```python
from build123d import *

# Parameters (mm, degrees)
SKETCH3_R                = 1.6
BOSS_EXTRUDE2_DEPTH      = 5
SKETCH8_W                = 6.531662429
SKETCH8_H                = 15.718756423
BOSS_EXTRUDE5_DEPTH      = 25.594989388
BOSS_EXTRUDE6_DEPTH      = 5
BOSS_EXTRUDE6_DEPTH_BACK = 15.725319597
BOSS_EXTRUDE7_DEPTH      = 15.715206985
FILLET3_R                = 6


with BuildPart() as part:
    # Sketch3 → Boss-Extrude2 (new body)
    with BuildSketch(Plane.XY):
        with BuildLine():
            Line((15.398328751, 23.358235096), (42.103650237, 35.3480109))
            ThreePointArc((42.103650237, 35.3480109), (43.812929052, 35.351800988), (44.957199874, 34.082040099))
            Line((44.957199874, 34.082040099), (42.962535727, 10.043789437))
            ThreePointArc((42.962535727, 10.043789437), (39.652134692, -17.353336053), (40.589325164, -44.933816726))
            Line((40.589325164, -44.933816726), (46.4215305, -44.933816726))
            Line((46.4215305, -44.933816726), (46.4215305, -60.652573149))
            Line((46.4215305, -60.652573149), (28.574574678, -60.652573149))
            ThreePointArc((28.574574678, -60.652573149), (27.026794649, -59.729266605), (26.047291344, -58.216424488))
            ThreePointArc((26.047291344, -58.216424488), (16.153529465, -18.922365583), (14.162802755, 21.549187347))
            ThreePointArc((14.162802755, 21.549187347), (14.525551977, 22.627878073), (15.398328751, 23.358235096))
        make_face()
        with Locations((17.26515434, 20.395199458)):
            Circle(SKETCH3_R, mode=Mode.SUBTRACT)
        with Locations((41.82515434, 31.625199458)):
            Circle(SKETCH3_R, mode=Mode.SUBTRACT)
        with Locations((39.04515434, 14.855199458)):
            Circle(SKETCH3_R, mode=Mode.SUBTRACT)
    extrude(amount=BOSS_EXTRUDE2_DEPTH)

    # Sketch8 → Boss-Extrude5 (add)
    with BuildSketch(Plane.XY.offset(5)):
        with Locations((43.155699286, -52.793194938)):
            Rectangle(SKETCH8_W, SKETCH8_H)
    extrude(amount=BOSS_EXTRUDE5_DEPTH)

    # Sketch9 → Boss-Extrude6 (add, two sides: drawn at the far end of the back side and taken through both)
    with BuildSketch(Plane(origin=(0, -44.933816726, 0), x_dir=(1, 0, 0), z_dir=(0, 1, 0)).offset(-BOSS_EXTRUDE6_DEPTH_BACK)):
        with BuildLine():
            Line((46.4215305, -30.594989388), (46.4215305, 0))
            Line((46.4215305, 0), (46.4215305, 2.879605598))
            Line((46.4215305, 2.879605598), (50.894134372, 2.879605598))
            ThreePointArc((50.894134372, 2.879605598), (48.34293367, -13.815617676), (46.4215305, -30.594989388))
        make_face()
    extrude(amount=BOSS_EXTRUDE6_DEPTH + BOSS_EXTRUDE6_DEPTH_BACK)

    # Sketch10 → Boss-Extrude7 (add)
    with BuildSketch(Plane(origin=(0, -44.933816726, 0), x_dir=(1, 0, 0), z_dir=(0, 1, 0))):
        with BuildLine():
            Line((29.146955031, -5), (41.859352304, -5))
            Line((41.859352304, -5), (41.859352304, -30.594989388))
            ThreePointArc((41.859352304, -30.594989388), (38.401030969, -16.358190815), (29.146955031, -5))
        make_face()
    extrude(amount=-BOSS_EXTRUDE7_DEPTH)

    # Fillet3
    # the kernel refuses this fillet: 6 mm, written as the material it adds along each edge
    with BuildSketch(Plane(origin=(46.4215305, -44.933816726, 30.594989388), x_dir=(0, 1, 0), z_dir=(0, 0, -1))) as fillet3_piece_1_section:
        with BuildLine():
            CenterArc((6, -5.916079783), FILLET3_R, 99.594068227, 80.405931773)
            Line((0, -5.916079783), (-0.12, -5.916079783))
            Line((-0.12, -5.916079783), (-0.12, 0))
            Line((-0.12, 0), (0, 0.12))
            ThreePointArc((0, 0.12), (2.5, 0.12), (4.98, 0.118321596))
            Line((4.98, 0.118321596), (5, 0))
        make_face()
    fillet3_piece_1 = extrude(amount=30.594989388, mode=Mode.PRIVATE)
    fillet3_piece_1 = fillet3_piece_1 - Plane(origin=(493.305440786, -43.701646152, 73.26789881), x_dir=(-0.9855086772136745, 0, -0.16962501919396705), z_dir=(0, -1, 0)) * Cylinder(448.916703265, 85, mode=Mode.PRIVATE)
    add(fillet3_piece_1)


solid = part.part
```
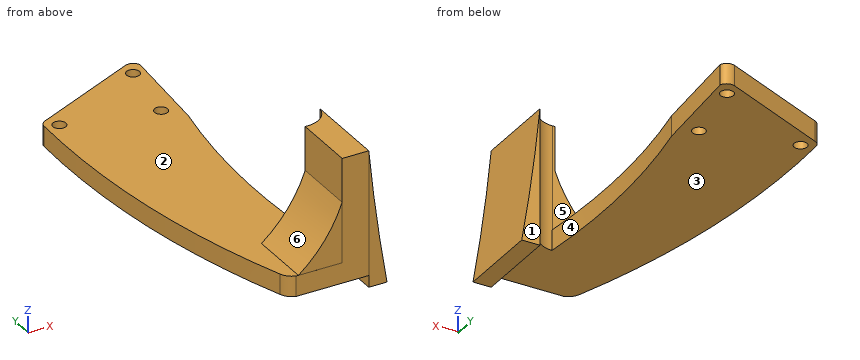
Input: part model. Units: mm. Frame: model coordinates. Face numbers are marked on the shaded views. A direction names the side the tool comes from. Round coordinates to 2 decimals unless told otherwise and drop trailing zeros. Loops run counter-clockwise (first coordinate to the right, second up) from the corner with the lowest first, then second, coordinate; pieces in that order, holes last.
1) Section query A-A on z = 1. Count the separate pieces of the cut face and the enclosed holes in it, plus the area to 3 significant figures.
Ans:
separate pieces: 1
enclosed holes: 3
area: 2,300 mm2
2) Pin query (flat end, axial travel): pin 1 (1.5 mm diameter, centred on x = 37, z = 10, fed in from -Y); pin 2 (5 mm diameter, centred on x = 41.83, y = 31.63, fed in from -Z); pin 3 (10 mm diameter, centred on x = 36, z = 3, fed in from -Y). Return the tip coordinate at first contact, or that it passes through.
Ans:
pin 1: stops at y = -60.65
pin 2: stops at z = 0
pin 3: stops at y = -60.65
3) Section query D-D on y = -51. Return the cut outline in (x, z), plus the area to 3 significant figures.
Ans:
outline: (23.6, 0) - (46.42, 0) - (46.42, -2.88) - (50.89, -2.88) arc R448.92 cw to (46.42, 30.59) - (39.89, 30.59) - (39.89, 19.84) arc R33.17 cw to (29.15, 5) - (23.6, 5) - close
area: 413 mm2
4) Set-up query: the marked faces 1, 2 and 3. Return all of +Z, -Z, +X, -X, +Y, -Y with unobstructed straight access to the full face (end or side cutting, diameter ignored); none if empty.
Ans:
face 1: +Z, -Z, +X, +Y
face 2: +Z, -X, +Y
face 3: -Z, -X, +Y, -Y
5) Pull-direction query (Y, two-part tool) for the marked faces 4, 5 and 6; classes: released by +Y, released by -Y, zero draft, split by the parting line, or undercut.
Ans:
face 4: undercut
face 5: released by +Y
face 6: zero draft
6) Material intervals for line 1 (Z direction, x = 20.5, y = 2.5); line 2 (Y direction, x = 40.5, z = 13); line 3 (Y direction, x = 48, z = 0), sorted ascending.
Ans:
line 1: z = 0 to 5
line 2: y = -60.65 to -44.93
line 3: y = -60.66 to -39.93
